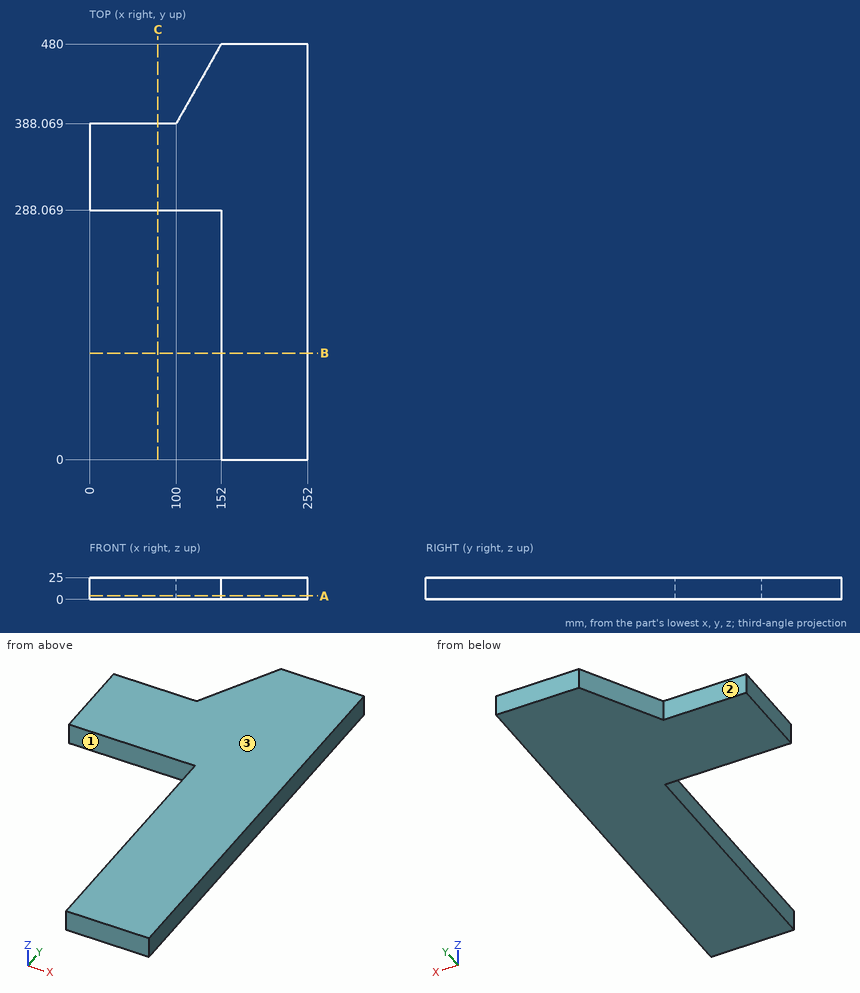
Study the drawing (mm; zero at the part's minimum x, y, z) and answer. A direction names the side the tool comes from. Coordinates: 2 decimals unless noted, no trailing zeros. Order: outer loops, then holes, each group sorted by start corner. A loop starts at its lowest first (then second) coordinate and runs counter-clockwise, first axis right, second up. Notation, with made-up numbers: (18, 15) -> (77, 15) arc R22 cw to (77, 51) -> close; hole circle Ø4 at (15, 83.5). An arc over 180 degrees is marked (long way). Answer in a Markdown table with one row per item. Add a question column.
Item 1: Find the intervals of material crossed by L1, parallel to Y at x = 40, z = 20.5; L2, parallel to X at y = 264.5, z = 2.75; L3, parallel to X at y = 400.5, z = 11.25, in increasing order. Write a range as from..to.
Item 2: Find section A-A (z = 4). Write down the section's boundary in (x, y).
Item 3: Find section B-B (y = 123). Write down the section's boundary in (x, z).
Item 4: Find section C-C (x = 79). Write down the section's boundary in (y, z).
Item 5: Which of the six approach directions +Z, -Z, +X, -X, +Y, -Y give full straight-line access (tool end or side, diameter ignored) to the marked faces 1, 2 and 3?
Item 6: Each of these flat-tipped pins is pushed along its axis until it touches: P1, Ø2, axis at x = 190, z = 20.5, coming from the -Y side; P2, Ø10, axis at x = 84.5, z = 21, coming from the +Y side; P3, Ø10, axis at x = 144.5, z = 10, coming from the -Y side. Where does it stop, or does it pass through?
Result set:
| question | item | result |
|---|---|---|
| 1 | L1 | y = 288.07..388.07 |
| 1 | L2 | x = 152..252 |
| 1 | L3 | x = 107.03..252 |
| 2 | outline | (0, 288.07) -> (152, 288.07) -> (152, 0) -> (252, 0) -> (252, 480) -> (152, 480) -> (100, 388.07) -> (0, 388.07) -> close |
| 3 | outline | (152, 0) -> (252, 0) -> (252, 25) -> (152, 25) -> close |
| 4 | outline | (288.07, 0) -> (388.07, 0) -> (388.07, 25) -> (288.07, 25) -> close |
| 5 | face 1 | +Z, -Z, -X, -Y |
| 5 | face 2 | +Z, -Z, -X, +Y |
| 5 | face 3 | +Z, +X, -X, +Y, -Y |
| 6 | P1 | stops at y = 0 |
| 6 | P2 | stops at y = 388.07 |
| 6 | P3 | stops at y = 288.07 |
